```python
from build123d import *

# Parameters (mm, degrees)
EXTRUDE_3_DEPTH     = 4.5
SKETCH_5_R          = 6.5
EXTRUDE_4_DEPTH     = 1
EXTRUDE_START       = -5.5
SKETCH_5_2_R        = 6.5
EXTRUDE_6_DEPTH     = 1
CUT_EXTRUDE_1_REACH = 13.258
CHAMFER_1_SIZE      = 0.2
FILLET_1_R          = 0.1


with BuildPart() as part:
    # 草图1 → 凸台-拉伸3 (new body)
    with BuildSketch(Plane.XY):
        with BuildLine():
            Line((0.973500707, 4.894118549), (1.037379867, 4.881412194))
            ThreePointArc((1.037379867, 4.881412194), (1.206083752, 4.765877122), (1.239075855, 4.564082984))
            Line((1.239075855, 4.564082984), (1.190890986, 4.368931892))
            ThreePointArc((1.190890986, 4.368931892), (1.544766642, 3.700642421), (2.258591893, 3.950226689))
            Line((2.258591893, 3.950226689), (2.351135088, 4.103452967))
            ThreePointArc((2.351135088, 4.103452967), (2.517154032, 4.222814031), (2.718141325, 4.185218003))
            Line((2.718141325, 4.185218003), (2.772295463, 4.149033365))
            Line((2.772295463, 4.149033365), (2.8264496, 4.112848728))
            ThreePointArc((2.8264496, 4.112848728), (2.938098308, 3.941548058), (2.891355764, 3.742489052))
            Line((2.891355764, 3.742489052), (2.77215766, 3.580632503))
            ThreePointArc((2.77215766, 3.580632503), (2.843352827, 2.827791189), (3.59835313, 2.785207889))
            Line((3.59835313, 2.785207889), (3.742489052, 2.891355764))
            ThreePointArc((3.742489052, 2.891355764), (3.941548058, 2.938098308), (4.112848728, 2.8264496))
            Line((4.112848728, 2.8264496), (4.149033365, 2.772295463))
            Line((4.149033365, 2.772295463), (4.185218003, 2.718141325))
            ThreePointArc((4.185218003, 2.718141325), (4.222814031, 2.517154032), (4.103452967, 2.351135088))
            Line((4.103452967, 2.351135088), (3.931388459, 2.247214275))
            ThreePointArc((3.931388459, 2.247214275), (3.709064318, 1.524434383), (4.390297723, 1.196166436))
            Line((4.390297723, 1.196166436), (4.564082984, 1.239075855))
            ThreePointArc((4.564082984, 1.239075855), (4.765877122, 1.206083752), (4.881412194, 1.037379867))
            Line((4.881412194, 1.037379867), (4.894118549, 0.973500707))
            Line((4.894118549, 0.973500707), (4.906824904, 0.909621546))
            ThreePointArc((4.906824904, 0.909621546), (4.864644598, 0.709546123), (4.690836654, 0.60184212))
            Line((4.690836654, 0.60184212), (4.492101004, 0.571678044))
            ThreePointArc((4.492101004, 0.571678044), (4.010104391, -0.011003739), (4.513859285, -0.574980514))
            Line((4.513859285, -0.574980514), (4.690836654, -0.60184212))
            ThreePointArc((4.690836654, -0.60184212), (4.864644598, -0.709546123), (4.906824904, -0.909621546))
            Line((4.906824904, -0.909621546), (4.894118549, -0.973500707))
            Line((4.894118549, -0.973500707), (4.881412194, -1.037379867))
            ThreePointArc((4.881412194, -1.037379867), (4.765877122, -1.206083752), (4.564082984, -1.239075855))
            Line((4.564082984, -1.239075855), (4.368931892, -1.190890986))
            ThreePointArc((4.368931892, -1.190890986), (3.700642421, -1.544766642), (3.950226689, -2.258591893))
            Line((3.950226689, -2.258591893), (4.103452967, -2.351135088))
            ThreePointArc((4.103452967, -2.351135088), (4.222814031, -2.517154032), (4.185218003, -2.718141325))
            Line((4.185218003, -2.718141325), (4.149033365, -2.772295463))
            Line((4.149033365, -2.772295463), (4.112848728, -2.8264496))
            ThreePointArc((4.112848728, -2.8264496), (3.941548058, -2.938098308), (3.742489052, -2.891355764))
            Line((3.742489052, -2.891355764), (3.580632503, -2.77215766))
            ThreePointArc((3.580632503, -2.77215766), (2.827791189, -2.843352827), (2.785207889, -3.59835313))
            Line((2.785207889, -3.59835313), (2.891355764, -3.742489052))
            ThreePointArc((2.891355764, -3.742489052), (2.938098308, -3.941548058), (2.8264496, -4.112848728))
            Line((2.8264496, -4.112848728), (2.772295463, -4.149033365))
            Line((2.772295463, -4.149033365), (2.718141325, -4.185218003))
            ThreePointArc((2.718141325, -4.185218003), (2.517154032, -4.222814031), (2.351135088, -4.103452967))
            Line((2.351135088, -4.103452967), (2.247214275, -3.931388459))
            ThreePointArc((2.247214275, -3.931388459), (1.524434383, -3.709064318), (1.196166436, -4.390297723))
            Line((1.196166436, -4.390297723), (1.239075855, -4.564082984))
            ThreePointArc((1.239075855, -4.564082984), (1.206083752, -4.765877122), (1.037379867, -4.881412194))
            Line((1.037379867, -4.881412194), (0.973500707, -4.894118549))
            Line((0.973500707, -4.894118549), (0.909621546, -4.906824904))
            ThreePointArc((0.909621546, -4.906824904), (0.709546123, -4.864644598), (0.60184212, -4.690836654))
            Line((0.60184212, -4.690836654), (0.571678044, -4.492101004))
            ThreePointArc((0.571678044, -4.492101004), (-0.011003739, -4.010104391), (-0.574980514, -4.513859285))
            Line((-0.574980514, -4.513859285), (-0.60184212, -4.690836654))
            ThreePointArc((-0.60184212, -4.690836654), (-0.709546123, -4.864644598), (-0.909621546, -4.906824904))
            Line((-0.909621546, -4.906824904), (-0.973500707, -4.894118549))
            Line((-0.973500707, -4.894118549), (-1.037379867, -4.881412194))
            ThreePointArc((-1.037379867, -4.881412194), (-1.206083752, -4.765877122), (-1.239075855, -4.564082984))
            Line((-1.239075855, -4.564082984), (-1.190890986, -4.368931892))
            ThreePointArc((-1.190890986, -4.368931892), (-1.544766642, -3.700642421), (-2.258591893, -3.950226689))
            Line((-2.258591893, -3.950226689), (-2.351135088, -4.103452967))
            ThreePointArc((-2.351135088, -4.103452967), (-2.517154032, -4.222814031), (-2.718141325, -4.185218003))
            Line((-2.718141325, -4.185218003), (-2.772295463, -4.149033365))
            Line((-2.772295463, -4.149033365), (-2.8264496, -4.112848728))
            ThreePointArc((-2.8264496, -4.112848728), (-2.938098308, -3.941548058), (-2.891355764, -3.742489052))
            Line((-2.891355764, -3.742489052), (-2.77215766, -3.580632503))
            ThreePointArc((-2.77215766, -3.580632503), (-2.843352827, -2.827791189), (-3.59835313, -2.785207889))
            Line((-3.59835313, -2.785207889), (-3.742489052, -2.891355764))
            ThreePointArc((-3.742489052, -2.891355764), (-3.941548058, -2.938098308), (-4.112848728, -2.8264496))
            Line((-4.112848728, -2.8264496), (-4.149033365, -2.772295463))
            Line((-4.149033365, -2.772295463), (-4.185218003, -2.718141325))
            ThreePointArc((-4.185218003, -2.718141325), (-4.222814031, -2.517154032), (-4.103452967, -2.351135088))
            Line((-4.103452967, -2.351135088), (-3.931388459, -2.247214275))
            ThreePointArc((-3.931388459, -2.247214275), (-3.709064318, -1.524434383), (-4.390297723, -1.196166436))
            Line((-4.390297723, -1.196166436), (-4.564082984, -1.239075855))
            ThreePointArc((-4.564082984, -1.239075855), (-4.765877122, -1.206083752), (-4.881412194, -1.037379867))
            Line((-4.881412194, -1.037379867), (-4.894118549, -0.973500707))
            Line((-4.894118549, -0.973500707), (-4.906824904, -0.909621546))
            ThreePointArc((-4.906824904, -0.909621546), (-4.864644598, -0.709546123), (-4.690836654, -0.60184212))
            Line((-4.690836654, -0.60184212), (-4.492101004, -0.571678044))
            ThreePointArc((-4.492101004, -0.571678044), (-4.010104391, 0.011003739), (-4.513859285, 0.574980514))
            Line((-4.513859285, 0.574980514), (-4.690836654, 0.60184212))
            ThreePointArc((-4.690836654, 0.60184212), (-4.864644598, 0.709546123), (-4.906824904, 0.909621546))
            Line((-4.906824904, 0.909621546), (-4.894118549, 0.973500707))
            Line((-4.894118549, 0.973500707), (-4.881412194, 1.037379867))
            ThreePointArc((-4.881412194, 1.037379867), (-4.765877122, 1.206083752), (-4.564082984, 1.239075855))
            Line((-4.564082984, 1.239075855), (-4.368931892, 1.190890986))
            ThreePointArc((-4.368931892, 1.190890986), (-3.700642421, 1.544766642), (-3.950226689, 2.258591893))
            Line((-3.950226689, 2.258591893), (-4.103452967, 2.351135088))
            ThreePointArc((-4.103452967, 2.351135088), (-4.222814031, 2.517154032), (-4.185218003, 2.718141325))
            Line((-4.185218003, 2.718141325), (-4.149033365, 2.772295463))
            Line((-4.149033365, 2.772295463), (-4.112848728, 2.8264496))
            ThreePointArc((-4.112848728, 2.8264496), (-3.941548058, 2.938098308), (-3.742489052, 2.891355764))
            Line((-3.742489052, 2.891355764), (-3.580632503, 2.77215766))
            ThreePointArc((-3.580632503, 2.77215766), (-2.827791189, 2.843352827), (-2.785207889, 3.59835313))
            Line((-2.785207889, 3.59835313), (-2.891355764, 3.742489052))
            ThreePointArc((-2.891355764, 3.742489052), (-2.938098308, 3.941548058), (-2.8264496, 4.112848728))
            Line((-2.8264496, 4.112848728), (-2.772295463, 4.149033365))
            Line((-2.772295463, 4.149033365), (-2.718141325, 4.185218003))
            ThreePointArc((-2.718141325, 4.185218003), (-2.517154032, 4.222814031), (-2.351135088, 4.103452967))
            Line((-2.351135088, 4.103452967), (-2.247214275, 3.931388459))
            ThreePointArc((-2.247214275, 3.931388459), (-1.524434383, 3.709064318), (-1.196166436, 4.390297723))
            Line((-1.196166436, 4.390297723), (-1.239075855, 4.564082984))
            ThreePointArc((-1.239075855, 4.564082984), (-1.206083752, 4.765877122), (-1.037379867, 4.881412194))
            Line((-1.037379867, 4.881412194), (-0.973500707, 4.894118549))
            Line((-0.973500707, 4.894118549), (-0.909621546, 4.906824904))
            ThreePointArc((-0.909621546, 4.906824904), (-0.709546123, 4.864644598), (-0.60184212, 4.690836654))
            Line((-0.60184212, 4.690836654), (-0.571678044, 4.492101004))
            ThreePointArc((-0.571678044, 4.492101004), (0.011003739, 4.010104391), (0.574980514, 4.513859285))
            Line((0.574980514, 4.513859285), (0.60184212, 4.690836654))
            ThreePointArc((0.60184212, 4.690836654), (0.709546123, 4.864644598), (0.909621546, 4.906824904))
            Line((0.909621546, 4.906824904), (0.973500707, 4.894118549))
        make_face()
    extrude(amount=EXTRUDE_3_DEPTH)

    # 草图5 → 凸台-拉伸4 (add)
    with BuildSketch(Plane.XY.offset(4.5)):
        Circle(SKETCH_5_R)
    extrude(amount=EXTRUDE_4_DEPTH)

    # 草图5<2> → 凸台-拉伸6 (add)
    with BuildSketch(Plane.XY.offset(4.5).offset(EXTRUDE_START)):
        Circle(SKETCH_5_2_R)
    extrude(amount=EXTRUDE_6_DEPTH)

    # 草图6 → 切除-拉伸1 (cut, up to next)
    with BuildSketch(Plane.XY.offset(5.5), mode=Mode.PRIVATE) as cut_extrude_1_sk1:
        with BuildLine():
            Line((-0.871779789, 1.8), (0.871779789, 1.8))
            ThreePointArc((0.871779789, 1.8), (0, -2), (-0.871779789, 1.8))
        make_face()
    cut_extrude_1_tool1 = extrude(cut_extrude_1_sk1.sketch, amount=-CUT_EXTRUDE_1_REACH, mode=Mode.PRIVATE) & part.part
    add(cut_extrude_1_tool1.solids().sort_by_distance((0, -0.035819, 5.5))[0], mode=Mode.SUBTRACT)

    # 倒角1
    chamfer_1_edges = [part.edges().sort_by_distance(p)[0] for p in [
        (0, -2, 5.5),
        (0, 1.8, 5.5),
        (0, 1.8, -1),
        (0, -2, -1),
    ]]
    chamfer(chamfer_1_edges, length=CHAMFER_1_SIZE)

    # 圆角1
    fillet_1_edges = [part.edges().sort_by_distance(p)[0] for p in [
        (-6.5, 0, 4.5),
        (-6.5, 0, 5.5),
        (-6.5, 0, 0),
        (-6.5, 0, -1),
    ]]
    fillet(fillet_1_edges, radius=FILLET_1_R)


solid = part.part
```
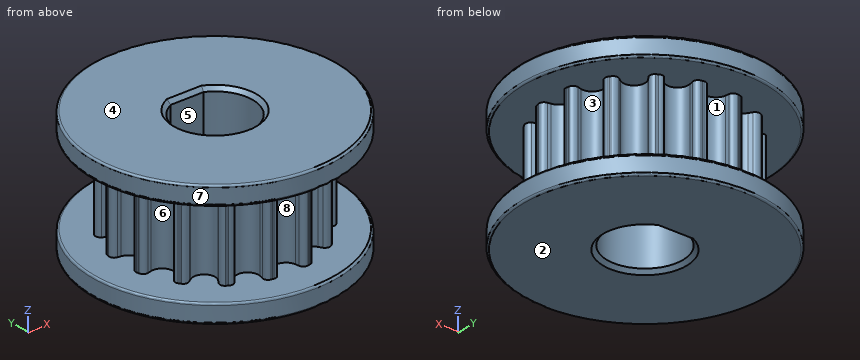
Could you check a few things on this model? Use its own coordinates, in mm. Face numbers are marked on the shaded views. A direction names the side the tool comes from. Coordinates: 2 decimals unless noted, no trailing zeros. Loops run counter-clockwise (first coordinate to the right, second up) from the corner with the lowest first, then second, coordinate; pieces in that order, holes last. Notation, with made-up numbers: M 79.5,21.25 L 112.5,21.25 A16 ccw 112.5,26.25 Z; hole C 49,-15.5 d1. An arc over 180 degrees is marked long. Put each result on its own line as item: value. Start each with the question number.
(1) Will these pins go through, and if not, where does the flat tip stop? P1, Ø0.5, axis at x = 0.5, z = 2, coming from the -Y side; P2, Ø1, axis at y = 3.5, z = 3.5, coming from the -X side; P3, Ø2.5, axis at x = 0, y = 0, coming from the +Z side; P4, Ø3, axis at x = -2, z = 2.5, coming from the +Y side.
(2) Suppose I cut it at B-B on x = 0. Please give me the cut outline in (y, z).
(3) For the marked faces 1, 2, 3, 4 and 5, which set-ups out of +Z, -Z, +X, -X, +Y, -Y let a thin tool reach every point of the face, with its end or its side?
(4) Thinking about a two-plate mould opening in Y: for the marked faces 6, 7 and 8, which applies, pulls with the +Y half, pulls with the -Y half, needs draft (parallel to the pull), parting line crosses it, or undercut?
(5) I need wall thicknesses on line 1 (Y direction, x = 0, z = 4.25); line 2 (Z direction, x = -4.25, y = -2.25); line 3 (X direction, y = 0, z = 1.75). Which ranges of each line are inside material? Lowest first, please. Write a range as from..to.
(6) Suppose I cut it at A-A on y = 0. Please give me the cut outline in (x, z), then the cut area to 3 significant figures.
Solutions:
1. P1: stops at y = -4.89
1. P2: stops at x = -2.94
1. P3: passes through
1. P4: stops at y = 4.91
2. outline: M -6.5,-0.9 A0.1 ccw -6.4,-1 L -2.2,-1 L -2,-0.8 L -2,5.3 L -2.2,5.5 L -6.4,5.5 A0.1 ccw -6.5,5.4 L -6.5,4.6 A0.1 ccw -6.4,4.5 L -4.01,4.5 L -4.01,0 L -6.4,0 A0.1 ccw -6.5,-0.1 Z; M 1.8,-0.8 L 2,-1 L 6.4,-1 A0.1 ccw 6.5,-0.9 L 6.5,-0.1 A0.1 ccw 6.4,0 L 4.01,0 L 4.01,4.5 L 6.4,4.5 A0.1 ccw 6.5,4.6 L 6.5,5.4 A0.1 ccw 6.4,5.5 L 2,5.5 L 1.8,5.3 Z
3. face 1: +Y
3. face 2: -Z, +X, -X, +Y, -Y
3. face 3: none
3. face 4: +Z, +X, -X, +Y, -Y
3. face 5: +Z, -Z
4. face 6: undercut
4. face 7: parting line crosses it
4. face 8: pulls with the -Y half
5. line 1: y = -4.01..-2, 1.8..4.01
5. line 2: z = -1..0, 4.5..5.5
5. line 3: x = -4.01..-2, 2..4.01
6. outline: M -6.5,-0.9 A0.1 ccw -6.4,-1 L -2.2,-1 L -2,-0.8 L -2,5.3 L -2.2,5.5 L -6.4,5.5 A0.1 ccw -6.5,5.4 L -6.5,4.6 A0.1 ccw -6.4,4.5 L -4.01,4.5 L -4.01,0 L -6.4,0 A0.1 ccw -6.5,-0.1 Z; M 2,-0.8 L 2.2,-1 L 6.4,-1 A0.1 ccw 6.5,-0.9 L 6.5,-0.1 A0.1 ccw 6.4,0 L 4.01,0 L 4.01,4.5 L 6.4,4.5 A0.1 ccw 6.5,4.6 L 6.5,5.4 A0.1 ccw 6.4,5.5 L 2.2,5.5 L 2,5.3 Z
6. area: 36.0 mm2
